Design review of the part built by this model. Coordinates are the model's own, in mm. Face numbers are marked on the shaded views. Coordinates: 2 decimals unless noted, no trailing zeros. Write each loop counter-clockwise with the first axis right and the second up, starting at its lowest first coordinate (ties: lowest second). Pieces come first, ordered by that corner, then holes.
Q1. Take a section at A-A (x = 70). Give the boundary of the cut face in (y, z).
Q2. Take a section at B-B (y = 0). Give the boundary of the cut face in (x, z), and give its area (3 significant figures).
Q3. Insertion check: pin 1 (1.8 mm diameter, centred on x = -105, y = 0, fed in from -Z). The pin has a flat end and moves straight along its axis. Give the tip position at first contact, or say it passes through.
Q4. For probe 1 along Y at (x, z) = (80, 1.85); probe 2 along Y at (x, z) = (-105, 1.95); probe 3 along X at (y, z) = (-1.75, 1), list the stretches that pass through material, from the lowest coordinate up.
Q5. Take a section at D-D (x = 105). Give the boundary of the cut face in (y, z).
Q6. Take a section at C-C (z = 2.05). Give the boundary of the cut face in (x, y), and give its area (3 significant figures).
Q7. Mouldability with a two-part tool opening along Z and no side actions: class the marked faces 1 and 2 as pulls with the +Z half, pulls with the -Z half, needs draft (parallel to the pull), parting line crosses it, or undercut.
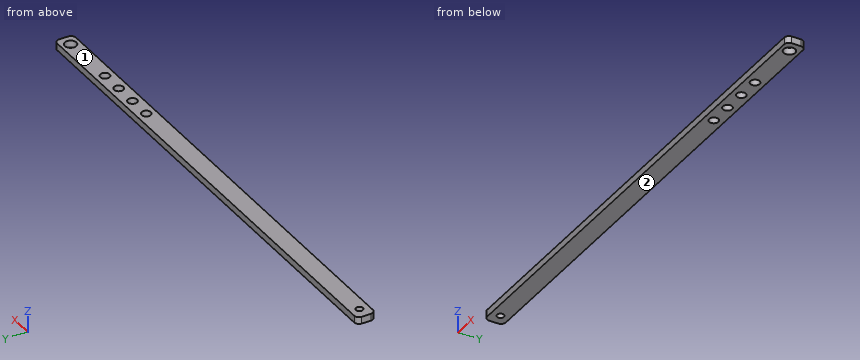
```python
from build123d import *

# Parameters (mm, degrees)
SKETCH1_W           = 220
SKETCH1_H           = 8
BOSS_EXTRUDE1_DEPTH = 3
FILLET1_R           = 2
SKETCH2_R           = 1.5
CUT_EXTRUDE1_DEPTH  = 3
SKETCH3_R           = 2.5
CUT_EXTRUDE2_DEPTH  = 3
SKETCH4_R           = 2
CUT_EXTRUDE3_DEPTH  = 3
LPATTERN1_COUNT     = 4
LPATTERN1_PITCH     = 10


with BuildPart() as part:
    # Sketch1 → Boss-Extrude1 (new body)
    with BuildSketch(Plane.XY):
        Rectangle(SKETCH1_W, SKETCH1_H)
    extrude(amount=BOSS_EXTRUDE1_DEPTH)

    # Fillet1
    fillet1_edges = [part.edges().sort_by_distance(p)[0] for p in [
        (110, -4, 1.5),
        (-110, -4, 1.5),
        (-110, 4, 1.5),
        (110, 4, 1.5),
    ]]
    fillet(fillet1_edges, radius=FILLET1_R)

    # Sketch2 → Cut-Extrude1 (cut)
    with BuildSketch(Plane.XY.offset(3)):
        with Locations((-105, 0)):
            Circle(SKETCH2_R)
    extrude(amount=-CUT_EXTRUDE1_DEPTH, mode=Mode.SUBTRACT)

    # Sketch3 → Cut-Extrude2 (cut)
    with BuildSketch(Plane.XY.offset(3)):
        with Locations((105, 0)):
            Circle(SKETCH3_R)
    extrude(amount=-CUT_EXTRUDE2_DEPTH, mode=Mode.SUBTRACT)

    # Sketch4 → Cut-Extrude3 (cut)
    with BuildSketch(Plane.XY.offset(3)):
        with Locations((80, 0)):
            Circle(SKETCH4_R)
    cut_extrude3 = extrude(amount=-CUT_EXTRUDE3_DEPTH, mode=Mode.SUBTRACT)

    # LPattern1: Cut-Extrude3 ×4
    with Locations(*[(-i * LPATTERN1_PITCH, 0, 0) for i in range(1, LPATTERN1_COUNT)]):
        add(cut_extrude3, mode=Mode.SUBTRACT)


solid = part.part
```
Response:
1. outline: (-4, 0) - (-2, 0) - (-2, 3) - (-4, 3) - close; (2, 0) - (4, 0) - (4, 3) - (2, 3) - close
2. outline: (-110, 0) - (-106.5, 0) - (-106.5, 3) - (-110, 3) - close; (-103.5, 0) - (48, 0) - (48, 3) - (-103.5, 3) - close; (52, 0) - (58, 0) - (58, 3) - (52, 3) - close; (62, 0) - (68, 0) - (68, 3) - (62, 3) - close; (72, 0) - (78, 0) - (78, 3) - (72, 3) - close; (82, 0) - (102.5, 0) - (102.5, 3) - (82, 3) - close; (107.5, 0) - (110, 0) - (110, 3) - (107.5, 3) - close
2. area: 588 mm2
3. pin 1: passes through
4. probe 1: y = -4 to -2, 2 to 4
4. probe 2: y = -4 to -1.5, 1.5 to 4
4. probe 3: x = -110 to 49.03, 50.97 to 59.03, 60.97 to 69.03, 70.97 to 79.03, 80.97 to 103.21, 106.79 to 110
5. outline: (-4, 0) - (-2.5, 0) - (-2.5, 3) - (-4, 3) - close; (2.5, 0) - (4, 0) - (4, 3) - (2.5, 3) - close
6. outline: (-110, -2) arc R2 ccw to (-108, -4) - (108, -4) arc R2 ccw to (110, -2) - (110, 2) arc R2 ccw to (108, 4) - (-108, 4) arc R2 ccw to (-110, 2) - close; hole circle Ø3 at (-105, 0); hole circle Ø4 at (50, 0); hole circle Ø4 at (60, 0); hole circle Ø4 at (70, 0); hole circle Ø4 at (80, 0); hole circle Ø5 at (105, 0)
6. area: 1,680 mm2
7. face 1: pulls with the +Z half
7. face 2: pulls with the -Z half
